Geometry: final body of the model. Coordinates: model frame, mm. Coordinates: 2 decimals unless noted, no trailing zeros. Loops run counter-clockwise (first coordinate to the right, second up) from the corner with the lowest first, then second, coordinate; pieces in that order, holes last. Notation, with made-up numbers: (-29, 60) - (22, 60) arc R23 cw to (22, 79) - close; hole circle Ø1 at (61, 32.25). An arc over 180 degrees is marked (long way). Answer in a Markdown table with one row per item.
Autodesk Inventor part; units mm, degrees
ref_plane "YZ Plane" through (0, 0, 0) normal (1, 0, 0) x (0, 1, 0)
ref_plane "XZ Plane" through (0, 0, 0) normal (0, 1, 0) x (-1, 0, 0)
ref_plane "XY Plane" through (0, 0, 0) normal (0, 0, 1) x (1, 0, 0)
sketch "Sketch1" plane through (0, 0, 0) normal (0, 1, 0) x (-1, 0, 0)
  line L0 (0, 17.4625) -> (0, 1.5875)
  line L1 (1.5875, 0) -> (17.4625, 0)
  line L2 (17.4625, 0) -> (17.4625, -1.5875)
  line L3 (17.4625, -1.5875) -> (-1.5875, -1.5875)
  line L4 (-1.5875, -1.5875) -> (-1.5875, 17.4625)
  line L5 (-1.5875, 17.4625) -> (0, 17.4625)
  arc A0 (0, 1.5875) -> (1.5875, 0) centre (1.5875, 1.5875) ccw
  point P0 (0, 0)
  dimension "d0" = 1.5875
  dimension "d1" = 19.05
  dimension "d2" = 1.5875
extrude "Extrusion1" add sketch "Sketch1" along normal blind 762
properties part number "Long Wall Cross" material "Aluminum 6061"
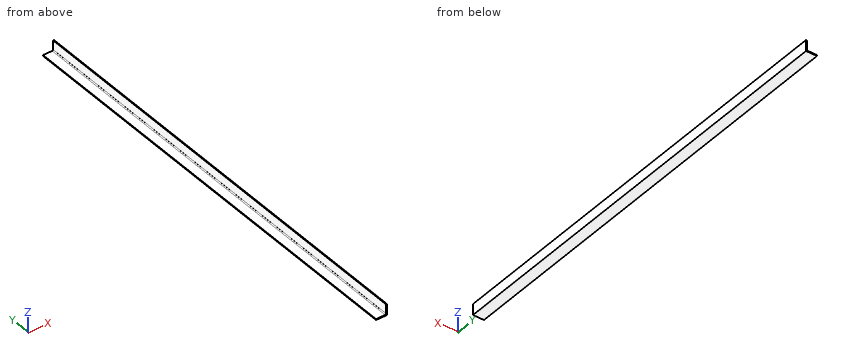
(1) Cut plane A-A on y = 458. Output: boundary loops of the cut face in (x, z) (1 decimal), then the cut area to 3 significant figures.
Verdict:
| item | result |
|---|---|
| outline | (-17.5, -1.6) - (1.6, -1.6) - (1.6, 17.5) - (0, 17.5) - (0, 1.6) arc R1.6 cw to (-1.6, 0) - (-17.5, 0) - close |
| area | 58.5 mm² |
(2) First-contact query: pin 1 Ø8 at (y, z) = (444, 12.5) entering from -X; pin 2 Ø8 at (x, y) = (-11.5, 436.5) entering from +Z. Flat tips, straight axial feed; report the tip coordinate or a pass-through.
Verdict:
| item | result |
|---|---|
| pin 1 | stops at x = 0 |
| pin 2 | stops at z = 0 |
(3) Cut plane C-C on z = 6.75. Output: boundary loops of the cut face in (x, y), then the cut area to 3 significant figures.
Verdict:
| item | result |
|---|---|
| outline | (0, 0) - (1.59, 0) - (1.59, 762) - (0, 762) - close |
| area | 1,210 mm² |
(4) Cut plane B-B on x = -10. Output: boundary loops of the cut face in (y, z), then the cut area to 3 significant figures.
Verdict:
| item | result |
|---|---|
| outline | (0, -1.59) - (762, -1.59) - (762, 0) - (0, 0) - close |
| area | 1,210 mm² |
(5) Ray query, probe 1 along Z at (x, y) = (-1.75, 456.5); probe 2 along Z at (x, y) = (-1, 455); probe 3 along X at (y, z) = (196, 15.5). Return the intervals inside material, ascending.
Verdict:
| item | result |
|---|---|
| probe 1 | z = -1.59 to 0 |
| probe 2 | z = -1.59 to 0.11 |
| probe 3 | x = 0 to 1.59 |
